Drawing for the job (mm, zero at the part's lowest x, y, z). A direction names the side the tool comes from. Round coordinates to 2 decimals unless told otherwise and drop trailing zeros. Write each loop counter-clockwise with the first axis right and the second up, starting at its lowest first coordinate (ties: lowest second). Pieces come first, ordered by that corner, then holes. Notation, with made-up numbers: (22.5, -36) -> (75.5, -36) arc R20 ccw to (75.5, -32) -> close; hole circle Ø8 at (20, -6). An arc over 180 degrees is marked (long way). Answer in a Markdown table with one row per item. Add a question column.
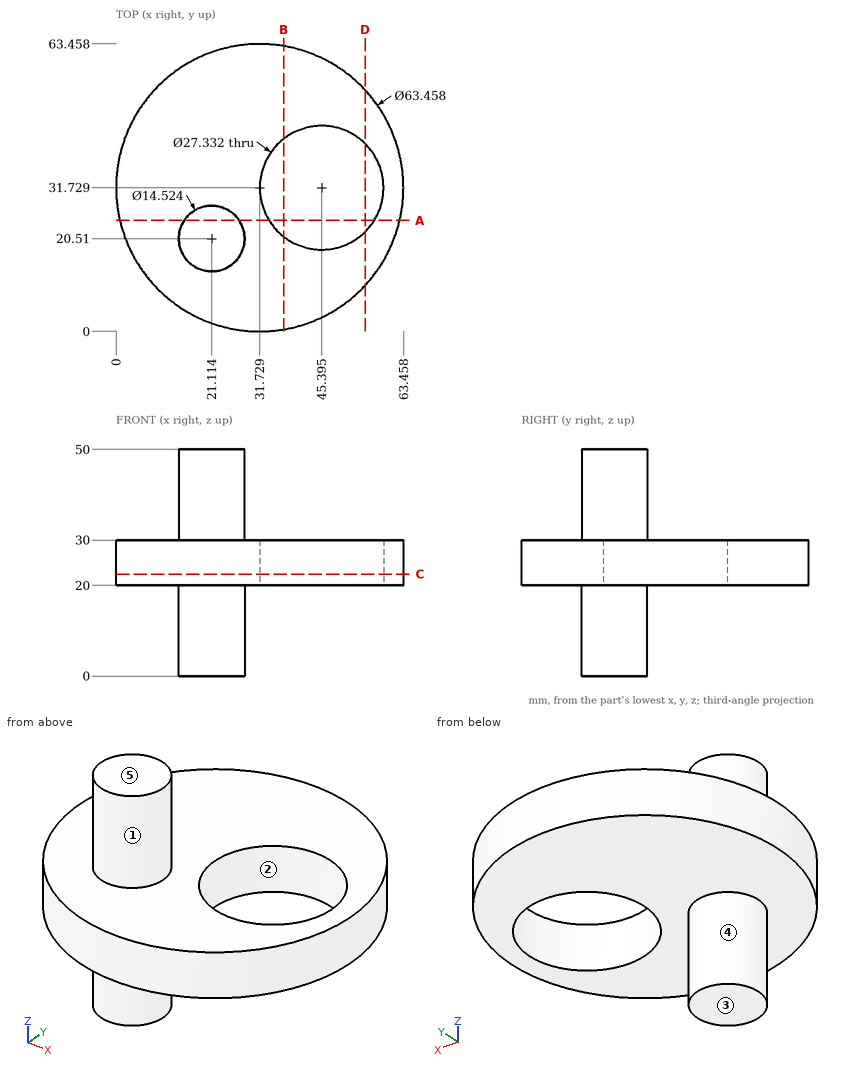
(1) Probe line 1 along Y through (x, z) = (21, 10); line 2 along Z through (x, y) = (7.5, 14); line 3 along Y through (x, z) = (53, 26.5) (1 decimal). List the from-to ranges inside material, lowest first.
(2) Drop flat-ended pins along their axis: P1, Ø19, axis at x = 40.5, y = 26, coming from the +Z side; P2, Ø5, axis at x = 42, y = 50.5, coming from the -Z side; P3, Ø10, axis at x = 12, z = 6, coming from the +Y side (1 decimal). Give the stop position or say it passes through.
(3) Mould opens along Y. For the marked faces 1, 2 and 3 say: pulls with the +Y half, pulls with the -Y half, needs draft (parallel to the pull), parting line crosses it, or undercut.
(4) Saw through at C-C (z = 22.5). List the corners of the cut face in (x, y) (1 decimal), plus the area to 3 significant figures.
(5) Which spindle directions (+Z, -Z, +X, -X, +Y, -Y) get a long thin tool onto all of the face, cutting with end or side? Do the marked faces 4 and 5. Say none if no direction does.
(6) Saw through at A-A (y = 24.5). List the corners of the cut face in (x, z) (1 decimal).
(7) Saw through at B-B (x = 37). List the corners of the cut face in (y, z) (1 decimal).
(8) Saw through at D-D (x = 55). List the corners of the cut face in (y, z), plus the area to 3 significant figures.
Answer sheet:
| question | item | result |
|---|---|---|
| 1 | line 1 | y = 13.25 to 27.77 |
| 1 | line 2 | z = 20 to 30 |
| 1 | line 3 | y = 8.2 to 20.4, 43.1 to 55.3 |
| 2 | P1 | stops at z = 30 |
| 2 | P2 | stops at z = 20 |
| 2 | P3 | stops at y = 26.5 |
| 3 | face 1 | parting line crosses it |
| 3 | face 2 | undercut |
| 3 | face 3 | needs draft |
| 4 | outline | circle Ø63.5 at (31.7, 31.7); hole circle Ø27.3 at (45.4, 31.7) |
| 4 | area | 2,580 mm² |
| 5 | face 4 | -Z |
| 5 | face 5 | +Z, +X, -X, +Y, -Y |
| 6 | outline | (0.8, 20) -> (15, 20) -> (15, 0) -> (27.2, 0) -> (27.2, 20) -> (33.8, 20) -> (33.8, 30) -> (27.2, 30) -> (27.2, 50) -> (15, 50) -> (15, 30) -> (0.8, 30) -> close; (57, 20) -> (62.6, 20) -> (62.6, 30) -> (57, 30) -> close |
| 7 | outline | (0.4, 20) -> (20.9, 20) -> (20.9, 30) -> (0.4, 30) -> close; (42.5, 20) -> (63, 20) -> (63, 30) -> (42.5, 30) -> close |
| 8 | outline | (10.16, 20) -> (22.01, 20) -> (22.01, 30) -> (10.16, 30) -> close; (41.45, 20) -> (53.3, 20) -> (53.3, 30) -> (41.45, 30) -> close |
| 8 | area | 237 mm² |
